For this review, take the finished solid that the model builds, in its own axes (mm). A direction names the side the tool comes from. Give positions to 0.01 mm unless a question says otherwise; leave off trailing zeros. Order: outer loops, then holes, each group sorted by start corner. A loop starts at its lowest first (then second) coordinate and runs counter-clockwise, first axis right, second up.
Item 1: For probe 1 along Z at (x, y) = (-10, -34); probe 2 along Z at (x, y) = (13.5, -10.5); probe 3 along Z at (x, y) = (26, -17), list the stretches that pass through material, from the lowest coordinate up.
Item 2: Machinability: for faces 4 (the cylindrical face through (-5, -15.6, 28.9)), 5 (the flat face through (3, -28, 18.6)), 6 (the cylindrical face through (-19.53, 21.55, 2.03)), which of the approach directions +Z, -Z, +X, -X, +Y, -Y give a long, thin tool a straight path to every point of the face, cutting with its end or side? Answer none if there is none.
Item 3: Consider section A-A (z = 22.5). Give the boundary of the cut face in (x, y).
Item 4: Consider section C-C (z = 35). Give the boundary of the cut face in (x, y), plus the area to 3 significant figures.
Item 5: The part is to be moulded in two halves that separate along Y. For faces 1 (the flat face through (0.1, -32.2, 23.8)), 2 (the cylindrical face through (26.29, -8.28, 18.99)), 3 (the cylindrical face through (20.79, -22.36, 2.03)), say which applies: released by +Y, released by -Y, zero draft, split by the parting line, or undercut.
Item 6: For P1, Ø8, axis at x = 7.5, y = 9.5, coming from the -Z side; P2, Ø6.5, axis at x = 18, z = 29.5, coming from the -Y side; P3, Ø4, axis at x = 5.5, z = 24.5, coming from the -Y side; P4, Ø1.8, axis at x = 20.86, y = 20.86, coming from the -Z side, all flat-tipped, find the tip position at first contact; note any pin that passes through.
Item 7: Consider section B-B (y = -5.5). Give the number of separate pieces and of enclosed holes in the cut face, plus the area to 3 significant figures.
Autodesk Inventor part; units mm, degrees
ref_plane "YZ Plane" through (0, 0, 0) normal (1, 0, 0) x (0, 1, 0)
ref_plane "XZ Plane" through (0, 0, 0) normal (0, 1, 0) x (-1, 0, 0)
ref_plane "XY Plane" through (0, 0, 0) normal (0, 0, 1) x (1, 0, 0)
sketch "Skizze1" plane through (0, 0, 0) normal (0, 0, 1) x (1, 0, 0)
  circle A0 centre (0, 0) radius 37.85
  dimension "d0" = 75.7
extrude "Extrusion1" add sketch "Skizze1" along normal blind 18.6
sketch "Skizze2" plane through (0, 0, 18.6) normal (0, 0, 1) x (1, 0, 0)
  circle A0 centre (0, 0) radius 37.85
  circle A1 centre (0, 0) radius 27.5647
extrude "Extrusion2" add sketch "Skizze2" along normal blind 0.8 contours A1
sketch "Skizze3" plane through (0, 0, 19.4) normal (0, 0, 1) x (1, 0, 0)
  circle A0 centre (0, 0) radius 27.5647
  circle A1 centre (0, 0) radius 36.25
  dimension "d5" = 72.5
extrude "Extrusion3" add sketch "Skizze3" along normal blind 21.4 contours A0 | A1
fillet "Rundung1" radius 12 1 edges at (-36.25, 0, 40.8)
sketch "Skizze4" plane through (0, 0, 0) normal (0, 1, 0) x (-1, 0, 0)
  line L0 (36.25, 28.8) -> (-36.25, 28.8)
  line L1 (23.5, 28.8) -> (-23.5, 28.8) construction
  line L2 (23.5, 33.8) -> (-23.5, 33.8)
  line L3 (-23.5, 23.8) -> (23.5, 23.8)
  arc A0 (23.5, 23.8) -> (23.5, 33.8) centre (23.5, 28.8) ccw
  arc A1 (-23.5, 33.8) -> (-23.5, 23.8) centre (-23.5, 28.8) ccw
  line L4 (0, -8.16) -> (0, 48.96) construction
  point P0 (0, 0)
  point P1 (0, 28.8)
  dimension "d9" = 10
  dimension "d10" = 47
extrude "Extrusion4" cut sketch "Skizze4" against normal through all
sketch "Skizze5" plane through (0, 0, 19.4) normal (0, 0, -1) x (-1, 0, 0)
  circle A0 centre (0, 0) radius 27.5647
  circle A1 centre (0, 0) radius 31.9541
extrude "Extrusion5" add sketch "Skizze5" against normal blind 15 contours A0 | A1
sketch "Skizze6" plane through (0, 0, 0) normal (0, 1, 0) x (-1, 0, 0)
  line L0 (40.5995, 28.8) -> (-50.4498, 28.8) construction
  line L1 (36.25, 19.4) -> (-36.25, 19.4) construction
  line L2 (0, -8.16) -> (0, 48.96) construction
  line L3 (23, 28.8) -> (9, 28.8) construction
  line L4 (23, 32.8) -> (9, 32.8)
  line L5 (9, 24.8) -> (23, 24.8)
  arc A0 (23, 24.8) -> (23, 32.8) centre (23, 28.8) ccw
  arc A1 (9, 32.8) -> (9, 24.8) centre (9, 28.8) ccw
  line L6 (-9, 28.8) -> (-23, 28.8) construction
  line L7 (-9, 32.8) -> (-23, 32.8)
  line L8 (-23, 24.8) -> (-9, 24.8)
  arc A2 (-9, 24.8) -> (-9, 32.8) centre (-9, 28.8) ccw
  arc A3 (-23, 32.8) -> (-23, 24.8) centre (-23, 28.8) ccw
  point P0 (0, 0)
  point P1 (16, 28.8)
  point P2 (-16, 28.8)
  dimension "d15" = 9.4
  dimension "d16" = 14
  dimension "d17" = 10
  dimension "d20" = 8
extrude "Extrusion6" cut sketch "Skizze6" against normal through all
sketch "Skizze7" plane through (0, 0, 0) normal (0, 0, -1) x (-1, 0, 0)
  circle A0 centre (0, 0) radius 29.5 construction
  line L0 (20.8597, 20.8597) -> (-20.8597, 20.8597) construction
  line L1 (-20.8597, 20.8597) -> (-20.8597, -20.8597) construction
  line L2 (-20.8597, -20.8597) -> (20.8597, -20.8597) construction
  line L3 (20.8597, -20.8597) -> (20.8597, 20.8597) construction
  line L4 (20.8597, 20.8597) -> (-20.8597, -20.8597) construction
  line L5 (-20.8597, 20.8597) -> (20.8597, -20.8597) construction
  dimension "d21" = 59
hole "Bohrung1" at (-20.8597, -20.8597, 0) at (20.8597, -20.8597, 0) at (20.8597, 20.8597, 0) at (-20.8597, 20.8597, 0) direction (0, 0, 1) diameter 3 depth 4 tip angle 118
properties part number "RPLidar A2" material "Kupfer, Guss"
Resolved:
1. probe 1: z = 0 to 18.6, 19.4 to 23.8
1. probe 2: z = 0 to 24.8, 32.8 to 40.8
1. probe 3: z = 0 to 18.6, 19.4 to 26.15, 31.45 to 38.68
2. face 4: -Y
2. face 5: none
2. face 6: -Z
3. outline: circle Ø72.5 at (0, 0)
4. outline: circle Ø69.05 at (0, 0)
4. area: 3,740 mm2
5. face 1: zero draft
5. face 2: split by the parting line
5. face 3: undercut
6. P1: stops at z = 0
6. P2: stops at y = 0
6. P3: stops at y = -36.07
6. P4: stops at z = 4.36
7. separate pieces: 1
7. enclosed holes: 2
7. area: 2,580 mm2
